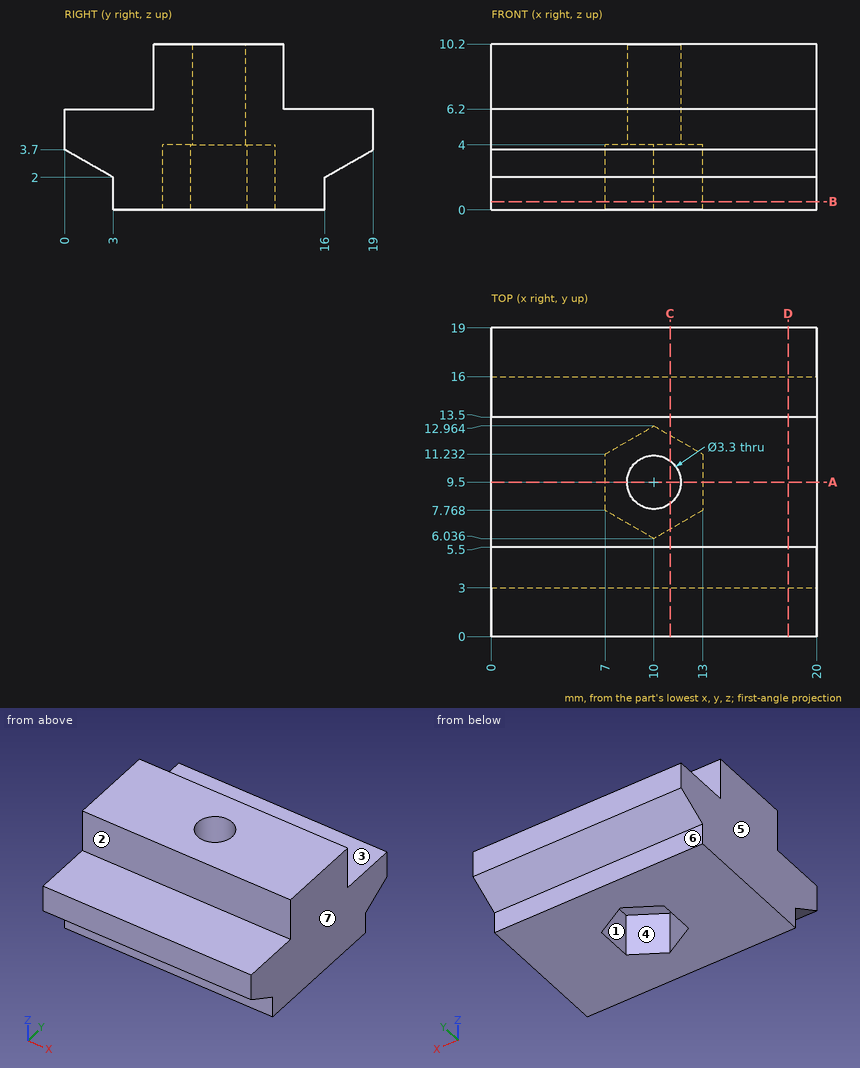
Study the drawing (mm; zero at the part's minimum x, y, z) and answer. A direction names the side the tool comes from. Round coordinates to 2 decimals unless told otherwise and drop trailing zeros. Order: outer loops, then holes, each group sorted by start corner. A loop starts at its lowest first (then second) coordinate and runs counter-clockwise, first axis right, second up. Notation, with made-up numbers: M 67,53 L 103,53 A20 ccw 103,64 Z; hole C 52.5,32 d9. An arc over 180 degrees is marked long. One line per item, written item: value.
Q1. Determine the mould class of the marked faces 4, 5, 6 and 7 for opening direction X: released by +X, released by -X, zero draft, split by the parting line, or undercut.
Derived:
face 4: undercut
face 5: released by -X
face 6: zero draft
face 7: released by +X
Q2. For the marked faces 1, 2 and 3, determine the directions among +Z, -Z, +X, -X, +Y, -Y from which every point of the face is accessible in a straight line to the end or side of a thin tool.
Derived:
face 1: -Z
face 2: +Z, +X, -X, -Y
face 3: +Z, +X, -X, +Y
Q3. Find section A-A on y = 9.5. Write down the section's boundary in (x, z).
Derived:
outline: M 0,0 L 7,0 L 7,4 L 8.35,4 L 8.35,10.2 L 0,10.2 Z; M 11.65,4 L 13,4 L 13,0 L 20,0 L 20,10.2 L 11.65,10.2 Z
Q4. Find section C-C on x = 11. Write down the section's boundary in (y, z), then the cut area to 3 significant figures.
Derived:
outline: M 0,3.7 L 3,2 L 3,0 L 6.61,0 L 6.61,4 L 8.19,4 L 8.19,10.2 L 5.5,10.2 L 5.5,6.2 L 0,6.2 Z; M 10.81,4 L 12.39,4 L 12.39,0 L 16,0 L 16,2 L 19,3.7 L 19,6.2 L 13.5,6.2 L 13.5,10.2 L 10.81,10.2 Z
area: 93.3 mm²
Q5. Flat-ended cylindrical pins translate along their axes: pin 1 (3 mm diameter, centred on x = 8, y = 16.5, fed in from +Z); pin 2 (4 mm diameter, centred on x = 8, z = 1.5, fed in from -Y); pin 3 (1 mm diameter, centred on x = 10, y = 11.5, fed in from -Z). Find the tip coordinate at first contact, or state that the pin passes through.
Derived:
pin 1: z = 6.2
pin 2: y = 0.35
pin 3: z = 4
Q6. Straight lines are drawn through the part: line 1 (X direction, y = 10.5, z = 3); line 2 (X direction, y = 9.5, z = 5.5); line 3 (Z direction, x = 8.25, y = 10.75). For each, find the intervals that lie inside material, in ascending order.
Derived:
line 1: 0 to 7, 13 to 20
line 2: 0 to 8.35, 11.65 to 20
line 3: 4 to 10.2
Q7. Find section D-D on x = 18.25. Write down the section's boundary in (y, z), then the cut area to 3 significant figures.
Derived:
outline: M 0,3.7 L 3,2 L 3,0 L 16,0 L 16,2 L 19,3.7 L 19,6.2 L 13.5,6.2 L 13.5,10.2 L 5.5,10.2 L 5.5,6.2 L 0,6.2 Z
area: 133 mm²
Q8. Find section B-B on z = 0.5. Write down the section's boundary in (x, y).
Derived:
outline: M 0,3 L 20,3 L 20,16 L 0,16 Z; hole M 7,7.77 L 10,6.04 L 13,7.77 L 13,11.23 L 10,12.96 L 7,11.23 Z
